```python
from build123d import *

# Parameters (mm, degrees)
EXTRUDE_1_DEPTH = 2


with BuildPart() as part:
    # 草图1 → 凸台-拉伸1 (new body)
    with BuildSketch(Plane.XY):
        with BuildLine():
            Line((0, 0), (235.10143352, 0))
            Line((235.10143352, 0), (235.10143352, 46.722315374))
            ThreePointArc((235.10143352, 46.722315374), (233.636967425, 50.25784928), (230.10143352, 51.722315374))
            Line((230.10143352, 51.722315374), (5, 51.722315374))
            ThreePointArc((5, 51.722315374), (1.464466094, 50.25784928), (0, 46.722315374))
            Line((0, 46.722315374), (0, 0))
        make_face()
        with BuildLine():
            Line((60.199702425, 42.318258034), (60.199702425, 22.318258034))
            ThreePointArc((60.199702425, 22.318258034), (62.55071676, 19.967243698), (64.901731095, 22.318258034))
            Line((64.901731095, 22.318258034), (64.901731095, 42.318258034))
            ThreePointArc((64.901731095, 42.318258034), (62.55071676, 44.669272369), (60.199702425, 42.318258034))
        make_face(mode=Mode.SUBTRACT)
        with BuildLine():
            Line((170.199702425, 42.318258034), (170.199702425, 22.318258034))
            ThreePointArc((170.199702425, 22.318258034), (172.55071676, 19.967243698), (174.901731095, 22.318258034))
            Line((174.901731095, 22.318258034), (174.901731095, 42.318258034))
            ThreePointArc((174.901731095, 42.318258034), (172.55071676, 44.669272369), (170.199702425, 42.318258034))
        make_face(mode=Mode.SUBTRACT)
    extrude(amount=EXTRUDE_1_DEPTH)


solid = part.part
```
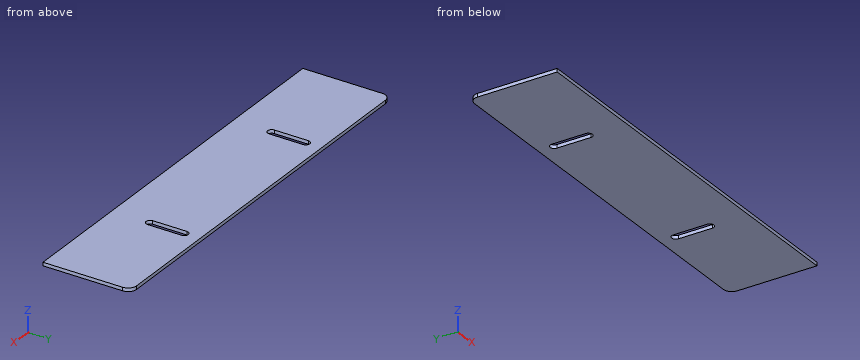
The model under review builds one solid part; all positions refer to its coordinate system, in mm. Give positions to 0.01 mm unless a question says otherwise; leave off trailing zeros. Loops run counter-clockwise (first coordinate to the right, second up) from the corner with the lowest first, then second, coordinate; pieces in that order, holes last. Notation, with made-up numbers: (17, 37.5) - (53, 37.5) arc R15 ccw to (53, 58.5) - close; hole circle Ø11 at (-28.75, 39). An arc over 180 degrees is marked (long way). Answer as a JSON object with one key per item and string values.
Q1. Add section A-A on y = 30. State the section outline as (x, z) points.
Worked out:
{"outline": "(0, 0) - (60.2, 0) - (60.2, 2) - (0, 2) - close; (64.9, 0) - (170.2, 0) - (170.2, 2) - (64.9, 2) - close; (174.9, 0) - (235.1, 0) - (235.1, 2) - (174.9, 2) - close"}
Q2. Add section B-B on z = 0.55. State the section outline as (x, y) points, plus the area to 3 significant figures.
Worked out:
{"outline": "(0, 0) - (235.1, 0) - (235.1, 46.72) arc R5 ccw to (230.1, 51.72) - (5, 51.72) arc R5 ccw to (0, 46.72) - close; hole (60.2, 22.32) arc R2.35 ccw to (64.9, 22.32) - (64.9, 42.32) arc R2.35 ccw to (60.2, 42.32) - close; hole (170.2, 22.32) arc R2.35 ccw to (174.9, 22.32) - (174.9, 42.32) arc R2.35 ccw to (170.2, 42.32) - close", "area": "11,900 mm^2"}
Q3. To check wall thickness, follow line 1 along X through (y, z) = (32, 1.2); line 2 along X through (y, z) = (21.5, 1); line 3 along X through (y, z) = (49.5, 1.9). State the ranges of each line that lie inside material, in increasing order.
Worked out:
{"line 1": "x = 0 to 60.2, 64.9 to 170.2, 174.9 to 235.1", "line 2": "x = 0 to 60.35, 64.75 to 170.35, 174.75 to 235.1", "line 3": "x = 0.84 to 234.26"}
